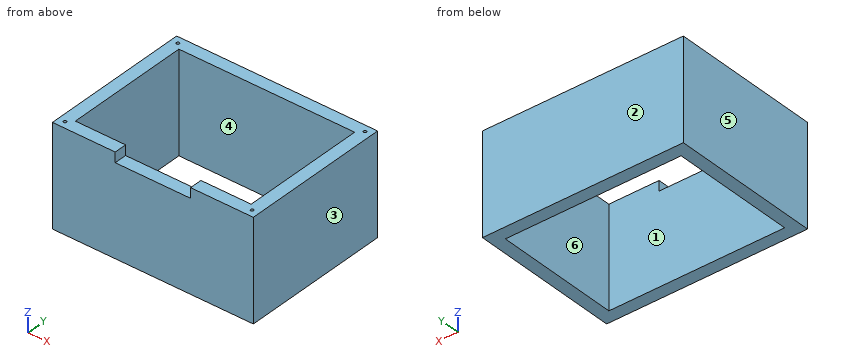
from build123d import *

# Parameters (mm, degrees)
SKETCH1_W           = 200
SKETCH1_H           = 150
BOSS_EXTRUDE1_DEPTH = 100
SKETCH2_W           = 175
SKETCH2_H           = 125
CUT_EXTRUDE1_DEPTH  = 100
SKETCH3_W           = 75
SKETCH3_H           = 10
CUT_EXTRUDE2_DEPTH  = 15
SKETCH4_R           = 1.5
CUT_EXTRUDE3_DEPTH  = 20


with BuildPart() as part:
    # Sketch1 → Boss-Extrude1 (new body)
    with BuildSketch(Plane.XY):
        with Locations((11.165128543, -17.619294273)):
            Rectangle(SKETCH1_W, SKETCH1_H)
    extrude(amount=BOSS_EXTRUDE1_DEPTH)

    # Sketch2 → Cut-Extrude1 (cut)
    with BuildSketch(Plane(origin=(0, 0, 0), x_dir=(-1, 0, 0), z_dir=(0, 0, -1))):
        with Locations((-11.165128543, -17.619294273)):
            Rectangle(SKETCH2_W, SKETCH2_H)
    extrude(amount=-CUT_EXTRUDE1_DEPTH, mode=Mode.SUBTRACT)

    # Sketch3 → Cut-Extrude2 (cut)
    with BuildSketch(Plane(origin=(0, -80.119294273, 0), x_dir=(1, 0, 0), z_dir=(0, 1, 0))):
        with Locations((11.165128543, -95)):
            Rectangle(SKETCH3_W, SKETCH3_H)
    extrude(amount=-CUT_EXTRUDE2_DEPTH, mode=Mode.SUBTRACT)

    # Sketch4 → Cut-Extrude3 (cut)
    with BuildSketch(Plane.XY.offset(100)):
        with Locations((-81.991725706, 50.537559977)):
            Circle(SKETCH4_R)
        with Locations((-81.991725706, -85.776148522)):
            Circle(SKETCH4_R)
        with Locations((104.321982793, 50.537559977)):
            Circle(SKETCH4_R)
        with Locations((104.321982793, -85.776148522)):
            Circle(SKETCH4_R)
    extrude(amount=-CUT_EXTRUDE3_DEPTH, mode=Mode.SUBTRACT)


solid = part.part
Read the model definition and answer for the solid it produces. Units are mm, in the model's axes. Face numbers are marked on the shaded views. A direction names the side the tool comes from. Round coordinates to 2 decimals unless told otherwise and drop trailing zeros. Write each loop counter-clockwise with the first axis right and the second up, starting at its lowest first coordinate (ties: lowest second). Pieces come first, ordered by that corner, then holes. Notation, with made-up numbers: (-40, -39) - (6, -39) arc R26 ccw to (6, -4) - close; hole circle Ø6 at (9.25, 54.5). An arc over 180 degrees is marked (long way). Use a Markdown table: item, result.
(1) The part is cut by section D-D (z = 86). Write down the section's boundary in (x, y), then the cut area to 3 significant figures.
Reported:
| item | result |
|---|---|
| outline | (-88.83, -92.62) - (111.17, -92.62) - (111.17, 57.38) - (-88.83, 57.38) - close; hole circle Ø3 at (-81.99, -85.78); hole circle Ø3 at (-81.99, 50.54); hole (-76.33, -80.12) - (98.67, -80.12) - (98.67, 44.88) - (-76.33, 44.88) - close; hole circle Ø3 at (104.32, -85.78); hole circle Ø3 at (104.32, 50.54) |
| area | 8,100 mm2 |
(2) The mould has two halves that part along X. Classify the marked faces 3, 4, 5 and 6: released by +X, released by -X, zero draft, split by the parting line, or undercut.
Reported:
| item | result |
|---|---|
| face 3 | released by +X |
| face 4 | undercut |
| face 5 | released by -X |
| face 6 | undercut |
(3) Straight lines are drawn through the part: line 1 along Y through (x, z) = (6, 28.5); line 2 along X through (y, z) = (-69, 91.5); line 3 along Y through (x, z) = (30, 94). For each, find the intervals that lie inside material, in ascending order. Write a range as [from, to].
Reported:
| item | result |
|---|---|
| line 1 | [-92.62, -80.12], [44.88, 57.38] |
| line 2 | [-88.83, -76.33], [98.67, 111.17] |
| line 3 | [44.88, 57.38] |
(4) Which of the six approach directions +Z, -Z, +X, -X, +Y, -Y give full straight-line access (tool end or side, diameter ignored) to the marked faces 1 and 2?
Reported:
| item | result |
|---|---|
| face 1 | +Z, -Z |
| face 2 | +Z, -Z, +X, -X, +Y |
(5) The part is cut by section B-B (x = -45.5). Write down the section's boundary in (y, z), then the cut area to 3 significant figures.
Reported:
| item | result |
|---|---|
| outline | (-92.62, 0) - (-80.12, 0) - (-80.12, 100) - (-92.62, 100) - close; (44.88, 0) - (57.38, 0) - (57.38, 100) - (44.88, 100) - close |
| area | 2,500 mm2 |
(6) The part is cut by section A-A (y = -56.5). Write down the section's boundary in (x, z).
Reported:
| item | result |
|---|---|
| outline | (-88.83, 0) - (-76.33, 0) - (-76.33, 100) - (-88.83, 100) - close; (98.67, 0) - (111.17, 0) - (111.17, 100) - (98.67, 100) - close |
(7) The part is cut by section C-C (z = 6). Write down the section's boundary in (x, y).
Reported:
| item | result |
|---|---|
| outline | (-88.83, -92.62) - (111.17, -92.62) - (111.17, 57.38) - (-88.83, 57.38) - close; hole (-76.33, -80.12) - (98.67, -80.12) - (98.67, 44.88) - (-76.33, 44.88) - close |
(8) Each of these flat-tipped pins is pushed along its axis until it touches: pin 1 Ø0.9 at (x, y) = (-82.5, -86) entering from +Z; pin 2 Ø4 at (x, y) = (8.5, -85.5) entering from +Z. Where does it stop, or does it pass through?
Reported:
| item | result |
|---|---|
| pin 1 | z = 80 |
| pin 2 | z = 90 |
